For this review, take the finished solid that the model builds, in its own axes (mm). A direction names the side the tool comes from. Coordinates: 2 decimals unless noted, no trailing zeros. Write each loop counter-clockwise with the first axis right and the second up, starting at its lowest first coordinate (ties: lowest second). Pieces come first, ordered by that corner, then holes. Notation, with made-up numbers: M -9,74.5 L 36,74.5 A18 cw 36,91.5 Z; hole C 24,47.25 d1. An arc over 180 degrees is marked long. Return JSON: item names as keys, results as strings.
Autodesk Inventor part; units mm, degrees
ref_plane "Work Plane1" through (0, 0, 10) normal (0, 0, 1) x (1, 0, 0)
ref_plane "Work Plane2" through (-40.9959, 0.8639, 22.2359) normal (0, 0, 1) x (1, 0, 0)
ref_plane "YZ Plane" through (0, 0, 0) normal (1, 0, 0) x (0, 1, 0)
ref_plane "Work Plane1" through (0, 0, 10) normal (0, 0, 1) x (1, 0, 0)
sketch "Sketch1" plane through (0, 0, 10) normal (0, 0, 1) x (1, 0, 0)
  line L0 (-4.0299, -0.3538) -> (-2.2322, 1.4439) construction
  arc A0 (-1.4439, 2.2322) -> (-2.2322, 1.4439) centre (-0.9299, 0.9299) ccw construction
  line L1 (-1.4439, 2.2322) -> (0.3538, 4.0299) construction
  line L2 (-37.8299, 42.2137) -> (-37.8299, 45.8299) construction
  line L3 (-37.8299, 45.8299) -> (-4.0299, 45.8299) construction
  line L4 (-4.0299, 45.8299) -> (-4.0299, 42.2137) construction
  line L5 (-4.0299, 4.0299) -> (0.3538, 4.0299)
  line L6 (-20.9299, 58.9723) -> (17.1124, 20.9299) construction
  line L7 (17.1124, 20.9299) -> (-20.9299, -17.1124) construction
  line L8 (-20.9299, -17.1124) -> (-58.9723, 20.9299) construction
  line L9 (-58.9723, 20.9299) -> (-20.9299, 58.9723) construction
  line L10 (-20.9299, 58.9723) -> (-20.9299, -17.1124) construction
  line L11 (17.1124, 20.9299) -> (-58.9723, 20.9299) construction
  line L12 (-20.9299, 58.9723) -> (32.8701, 58.9723) construction
  line L13 (-43.4299, 43.4299) -> (1.5701, 43.4299) construction
  line L14 (1.5701, 43.4299) -> (1.5701, -1.5701) construction
  line L15 (1.5701, -1.5701) -> (-43.4299, -1.5701) construction
  line L16 (-43.4299, -1.5701) -> (-43.4299, 43.4299) construction
  line L17 (-43.4299, 43.4299) -> (1.5701, -1.5701) construction
  line L18 (1.5701, 43.4299) -> (-43.4299, -1.5701) construction
  line L19 (-43.4299, 5.3876) -> (-43.4299, 36.4723)
  line L20 (-43.4299, 36.4723) -> (-36.4723, 43.4299)
  line L21 (-36.4723, 43.4299) -> (-5.3876, 43.4299)
  line L22 (-5.3876, 43.4299) -> (1.5701, 36.4723)
  line L23 (1.5701, 36.4723) -> (1.5701, 5.3876)
  line L24 (1.5701, 5.3876) -> (-5.3876, -1.5701)
  line L25 (-5.3876, -1.5701) -> (-36.4723, -1.5701)
  line L26 (-36.4723, -1.5701) -> (-43.4299, 5.3876)
  line L27 (-4.0299, 42.2137) -> (-37.8299, 42.2137)
  line L28 (-4.0299, -0.3538) -> (-4.0299, 4.0299)
  circle A1 centre (-20.9299, 20.9299) radius 11.75
  point P0 (-37.8299, 4.0299)
  dimension "d18" = 53.8
  dimension "d19" = 45
  dimension "d20" = 53.8
  dimension "d21" = 45
  dimension "d22" = 45
  dimension "d30" = 23.5
extrude "Extrusion1" add sketch "Sketch1" along normal blind 5 contours L28 L24 L25 L26 L19 L20 L27 L22 L23 L5 | L5 L24 L28 | L27 L20 L21 L22 | A1
ref_plane "Work Plane2" through (-40.9959, 0.8639, 22.2359) normal (0, 0, 1) x (1, 0, 0)
sketch "Sketch3" plane through (0, 0, 10) normal (0, 0, -1) x (-1, 0, 0)
  line L0 (37.8299, -0.4701) -> (37.8299, 4.0299) construction
  line L1 (4.0299, 4.0299) -> (4.0299, -0.4701) construction
  line L2 (37.8299, -0.4701) -> (37.8299, 1.1886) construction
  line L3 (4.0299, -3.9701) -> (4.0299, -0.3538) construction
  line L4 (45.8299, 4.0299) -> (42.2137, 4.0299) construction
  line L5 (-0.3538, 4.0299) -> (-3.9701, 4.0299) construction
  line L6 (-3.9701, 37.8299) -> (-0.3538, 37.8299) construction
  line L7 (4.0299, 42.2137) -> (4.0299, 45.8299) construction
  line L8 (37.8299, 45.8299) -> (37.8299, 42.2137) construction
  line L9 (42.2137, 37.8299) -> (45.8299, 37.8299) construction
  line L10 (37.8299, 37.7299) -> (45.8299, 37.7299)
  line L11 (45.8299, 37.7299) -> (45.8299, 4.1299)
  line L12 (45.8299, 4.1299) -> (37.8299, 4.1299)
  line L13 (37.8299, 4.1299) -> (37.8299, 37.7299)
  line L14 (37.7299, 4.0299) -> (4.1299, 4.0299)
  line L15 (4.1299, 4.0299) -> (4.1299, -3.9701)
  line L16 (4.1299, -3.9701) -> (37.7299, -3.9701)
  line L17 (37.7299, -3.9701) -> (37.7299, 4.0299)
  line L18 (4.0299, 4.1299) -> (-3.9701, 4.1299)
  line L19 (-3.9701, 4.1299) -> (-3.9701, 37.7299)
  line L20 (-3.9701, 37.7299) -> (4.0299, 37.7299)
  line L21 (4.0299, 37.7299) -> (4.0299, 4.1299)
  line L22 (4.1299, 37.8299) -> (37.7299, 37.8299)
  line L23 (37.7299, 37.8299) -> (37.7299, 45.8299)
  line L24 (37.7299, 45.8299) -> (4.1299, 45.8299)
  line L25 (4.1299, 45.8299) -> (4.1299, 37.8299)
  point P0 (0, 0)
  dimension "d23" = 0.1
  dimension "d24" = 0.1
  dimension "d25" = 0.1
  dimension "d26" = 0.1
  dimension "d27" = 0.1
extrude "Extrusion3" add sketch "Sketch3" against normal up to surface (5 mm away)
sketch "Sketch6" plane through (0, 0, 15) normal (0, 0, 1) x (1, 0, 0)
  line L0 (-37.7299, 45.8299) -> (-4.1299, 45.8299)
  line L1 (3.9701, 37.7299) -> (3.9701, 4.1299)
  point P0 (0, 0)
  point P1 (-20.9299, 20.9299)
  point P2 (-20.9299, 45.8299)
  point P3 (3.9701, 20.9299)
hole "Hole1" at (-20.9299, 20.9299, 15) direction (0, 0, -1) diameter 1 depth 8 countersink diameter 6 countersink angle 90
properties part number "20_Cube_Insert_Pinhole_conic hole"
1. For faces 1 (the face through (-44, 37.73, 12)), 2 (the face through (-4.13, 44, 12)), 3 (the face through (-44, 4.13, 12)), list the 3-axis set-ups (+Z, -Z, +X, -X, +Y, -Y) from which the entire face can be reached by the end or side of a thin tool; tool diameter is ignored.
Checks:
{"face 1": "+Z, -Z, -X, +Y", "face 2": "+Z, -Z, +X, +Y", "face 3": "+Z, -Z, -X, -Y"}
2. Clearance check with flat-ended pins moving along their axes: pin 1 Ø1.1 at (y, z) = (-3, 13) entering from +X; pin 2 Ø3 at (y, z) = (-2.5, 13.5) entering from -X; pin 3 Ø1.8 at (x, z) = (1.5, 11.5) entering from +Y. State where each tip first meets the part, or that it passes through.
Checks:
{"pin 1": "x = -4.13", "pin 2": "x = -37.73", "pin 3": "y = 37.73"}
3. We need section B-B (y = 40). State the section outline as (x, z) points.
Checks:
{"outline": "M -39.9,10 L -1.96,10 L -1.96,15 L -39.9,15 Z"}
4. We need section C-C (x = -41). State the section outline as (y, z) points.
Checks:
{"outline": "M 2.96,10 L 38.9,10 L 38.9,15 L 2.96,15 Z"}
5. We need section A-A (z = 13.1). State the section outline as (x, y) points, plus the area to 3 significant figures.
Checks:
{"outline": "M -45.83,4.13 L -42.17,4.13 L -37.73,-0.31 L -37.73,-3.97 L -4.13,-3.97 L -4.13,-0.31 L 0.31,4.13 L 3.97,4.13 L 3.97,37.73 L 0.31,37.73 L -4.13,42.17 L -4.13,45.83 L -37.73,45.83 L -37.73,42.17 L -42.17,37.73 L -45.83,37.73 Z; hole C -20.93,20.93 d2.2", "area": "2,250 mm2"}
6. Draft analysis for pull direction Y (two halves, no side actions). For faces 4 (the face through (-21.84, 21.13, 12.93)), 5 (the face through (-1.94, 39.98, 12.46)), 6 (the face through (-21, 16, 10)), state which applies: +Y half, -Y half, draft (parallel to the pull), parting line (faces both ways), or undercut.
Checks:
{"face 4": "undercut", "face 5": "+Y half", "face 6": "draft"}
7. Wall thickness on L1, parallel to Y at x = 0.5, z = 12.6; L2, parallel to X at y = 1, z = 10.3; L3, parallel to Z at x = -21, y = 22: over which ranges is each line inside the solid? List them lowest first. Write a range as from..to.
Checks:
{"L1": "4.13..37.73", "L2": "-39.04..-2.82", "L3": "10..13.07"}
